Geometry: see drawing. Coordinates: mm, zero at the bounding-box minimum. A direction names the side the tool comes from. Coordinates: 2 decimals unless noted, no trailing zeros. Order: outer loops, then holes, each group sorted by start corner. A loop starts at its lowest first (then second) coordinate and runs counter-clockwise, first axis right, second up.
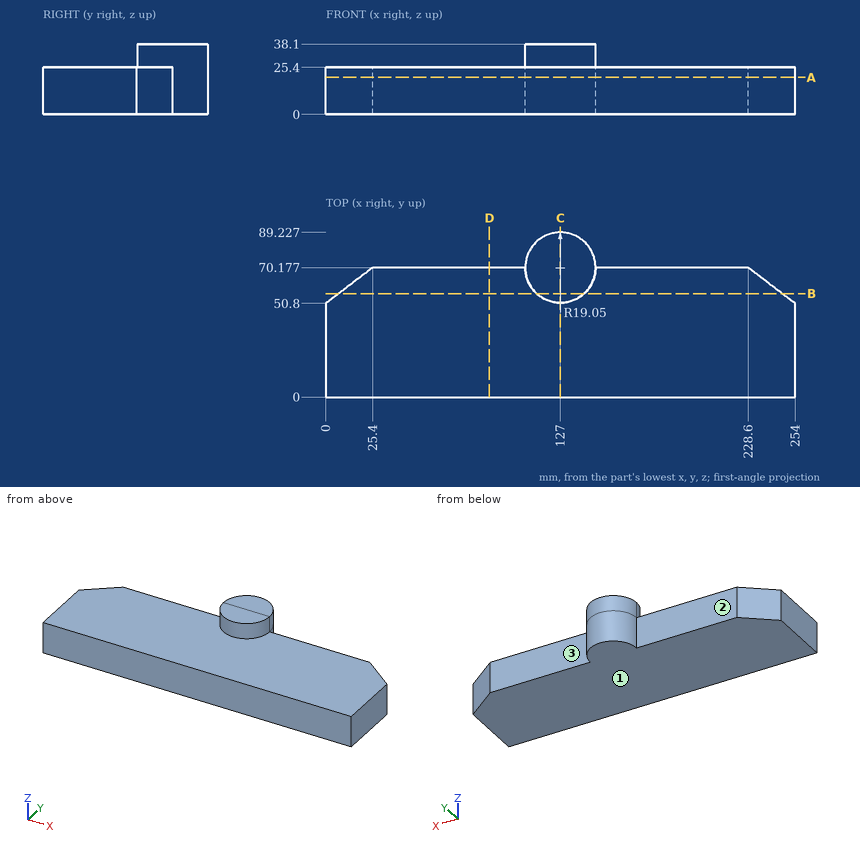
Item 1: Cut plane D-D on x = 88.5. Return loops of the section in (y, z).
Response values:
outline: (0, 0) - (70.18, 0) - (70.18, 25.4) - (0, 25.4) - close
Item 2: Cut plane C-C on x = 127. Return loops of the section in (y, z), then the cut area to 3 significant figures.
Response values:
outline: (0, 0) - (89.23, 0) - (89.23, 38.1) - (51.13, 38.1) - (51.13, 25.4) - (0, 25.4) - close
area: 2,750 mm2
Item 3: Pin query (flat end, axial travel): pin 1 Ø4 at (x, y) = (184, 20) entering from +Z; pin 2 Ø10 at (x, z) = (83.5, 4) entering from +Y; pin 3 Ø1 at (x, y) = (228, 41.5) entering from -Z; pin 4 Ø12 at (y, z) = (65, 11.5) entering from -X. Return the tip coordinate at first contact, or that it passes through.
Response values:
pin 1: stops at z = 25.4
pin 2: stops at y = 70.18
pin 3: stops at z = 0
pin 4: stops at x = 10.75
Item 4: Access query for the marked faces 1, 2 and 3. Directions: +Z, -Z, +X, -X, +Y, -Y. A direction counts if a zero-diameter tool reaches every point of the face in a straight line with its end or side. Return the directions, or none.
Response values:
face 1: -Z, +X, -X, +Y, -Y
face 2: +Z, -Z, -X, +Y
face 3: +Z, -Z, +X, +Y
Item 5: Cut plane A-A on z = 20. Return loops of the section in (x, y), then the cut area to 3 significant figures.
Response values:
outline: (0, 0) - (254, 0) - (254, 50.8) - (228.6, 70.18) - (146.05, 70.18) arc R19.05 ccw to (107.95, 70.18) - (25.4, 70.18) - (0, 50.8) - close
area: 17,900 mm2
Item 6: Ray query, probe 1 along Y at (x, z) = (226, 14.5); probe 2 along Z at (x, y) = (20, 61); probe 3 along X at (y, z) = (71, 6). Return the intervals inside material, ascending.
Response values:
probe 1: y = 0 to 70.18
probe 2: z = 0 to 25.4
probe 3: x = 107.97 to 146.03
Item 7: Cut plane B-B on y = 56. Return loops of the section in (x, z) (1 decimal).
Response values:
outline: (6.8, 0) - (247.2, 0) - (247.2, 25.4) - (139.7, 25.4) - (139.7, 38.1) - (114.3, 38.1) - (114.3, 25.4) - (6.8, 25.4) - close
